The model under review builds one solid part; all positions refer to its coordinate system, in mm. A direction names the side the tool comes from. Coordinates: 2 decimals unless noted, no trailing zeros. Order: outer loops, then holes, each group sorted by start corner. A loop starts at its lowest first (then second) coordinate and runs counter-clockwise, first axis right, second up.
Autodesk Inventor part; units mm, degrees
ref_plane "YZ Plane" through (0, 0, 0) normal (1, 0, 0) x (0, 1, 0)
ref_plane "XZ Plane" through (0, 0, 0) normal (0, 1, 0) x (-1, 0, 0)
ref_plane "XY Plane" through (0, 0, 0) normal (0, 0, 1) x (1, 0, 0)
sketch "CONTOURS" plane through (0, 0, 0) normal (0, 0, 1) x (1, 0, 0)
  line L0 (1512.926, 262.3244) -> (1483.7011, 302.5491)
  arc A0 (1490.3116, 325.9808) -> (1483.7011, 302.5491) centre (1496.2408, 311.6597) ccw
  line L1 (1490.3116, 325.9808) -> (1515.055, 336.2252)
  arc A1 (1515.055, 336.2252) -> (1520.7765, 358.748) centre (1509.5083, 349.6224) ccw
  line L2 (1520.7765, 358.748) -> (1420.6454, 482.3882)
  arc A2 (1420.6454, 482.3882) -> (1397.875, 482.0914) centre (1409.3772, 473.2625) ccw
  line L3 (1397.875, 482.0914) -> (1387.5892, 468.6913)
  arc A3 (1362.754, 469.0184) -> (1387.5892, 468.6913) centre (1375.2938, 478.1291) ccw
  line L4 (1362.754, 469.0184) -> (1334.3843, 508.066)
  arc A4 (193.4245, 508.066) -> (1334.3843, 508.066) centre (763.9044, 1294.3771) ccw
  line L5 (193.4245, 508.066) -> (165.0547, 469.0184)
  arc A5 (165.0547, 469.0184) -> (171.943, 446.828) centre (176.7854, 460.4955) ccw
  line L6 (171.943, 446.828) -> (187.8658, 441.1866)
  arc A6 (195.6892, 418.1351) -> (187.8658, 441.1866) centre (182.6894, 426.5765) ccw
  line L7 (195.6892, 418.1351) -> (109.0426, 284.6979)
  arc A7 (84.2549, 283.0747) -> (109.0426, 284.6979) centre (96.0429, 293.1392) ccw
  line L8 (84.2549, 283.0747) -> (66.8658, 303.4414)
  arc A8 (66.8658, 303.4414) -> (44.1076, 302.5491) centre (55.8384, 294.0262) ccw
  line L9 (44.1076, 302.5491) -> (14.8827, 262.3244)
  arc A9 (14.8827, 262.3244) -> (1512.926, 262.3244) centre (763.9044, 1294.1149) ccw
sketch "HOLES" plane through (0, 0, 0) normal (0, 0, 1) x (1, 0, 0)
  line L0 (224.6944, 455.9957) -> (218.4625, 446.9313)
  arc A0 (212.9002, 445.9014) -> (218.4625, 446.9313) centre (215.1664, 449.1975) ccw
  line L1 (212.9002, 445.9014) -> (183.2349, 466.2968)
  arc A1 (182.205, 471.8591) -> (183.2349, 466.2968) centre (185.5011, 469.5929) ccw
  line L2 (182.205, 471.8591) -> (188.4369, 480.9234)
  arc A2 (193.9992, 481.9534) -> (188.4369, 480.9234) centre (191.733, 478.6573) ccw
  line L3 (193.9992, 481.9534) -> (223.6644, 461.558)
  arc A3 (224.6944, 455.9957) -> (223.6644, 461.558) centre (221.3983, 458.2619) ccw
  line L4 (87.0245, 255.754) -> (80.7926, 246.6896)
  arc A4 (75.2303, 245.6596) -> (80.7926, 246.6896) centre (77.4965, 248.9557) ccw
  line L5 (75.2303, 245.6596) -> (45.5651, 266.055)
  arc A5 (44.5351, 271.6173) -> (45.5651, 266.055) centre (47.8312, 269.3511) ccw
  line L6 (44.5351, 271.6173) -> (50.767, 280.6817)
  arc A6 (56.3293, 281.7117) -> (50.767, 280.6817) centre (54.0631, 278.4155) ccw
  line L7 (56.3293, 281.7117) -> (85.9946, 261.3163)
  arc A7 (87.0245, 255.754) -> (85.9946, 261.3163) centre (83.7284, 258.0201) ccw
  line L8 (1487.4439, 359.9016) -> (1478.716, 353.2066)
  arc A8 (1473.1076, 353.9459) -> (1478.716, 353.2066) centre (1476.2814, 356.3804) ccw
  line L9 (1473.1076, 353.9459) -> (1406.7666, 440.4321)
  arc A9 (1407.5058, 446.0405) -> (1406.7666, 440.4321) centre (1409.9404, 442.8667) ccw
  line L10 (1407.5058, 446.0405) -> (1416.2338, 452.7354)
  arc A10 (1421.8421, 451.9962) -> (1416.2338, 452.7354) centre (1418.6683, 449.5616) ccw
  line L11 (1421.8421, 451.9962) -> (1488.1832, 365.51)
  arc A11 (1487.4439, 359.9016) -> (1488.1832, 365.51) centre (1485.0094, 363.0754) ccw
sketch "LETTERS" plane through (0, 0, 0) normal (0, 0, 1) x (1, 0, 0)
  line L0 (221.0345, 299.5651) -> (214.0787, 303.3807)
  line L1 (214.0787, 303.3807) -> (223.8436, 320.6336)
  line L2 (223.8436, 320.6336) -> (229.7881, 317.2691)
  line L3 (232.463, 314.1509) -> (232.5322, 313.9591)
  line L4 (232.5322, 313.9591) -> (232.5968, 313.7631)
  line L5 (232.5968, 313.7631) -> (232.6568, 313.5633)
  line L6 (232.6568, 313.5633) -> (232.7121, 313.3597)
  line L7 (232.7121, 313.3597) -> (232.7625, 313.1525)
  line L8 (232.7625, 313.1525) -> (232.8082, 312.942)
  line L9 (232.8082, 312.942) -> (232.8489, 312.7282)
  line L10 (232.8489, 312.7282) -> (232.8846, 312.5116)
  line L11 (232.8846, 312.5116) -> (232.9153, 312.2921)
  line L12 (232.9153, 312.2921) -> (232.941, 312.0702)
  line L13 (232.941, 312.0702) -> (232.9616, 311.8459)
  line L14 (232.9616, 311.8459) -> (232.9772, 311.6196)
  line L15 (232.9772, 311.6196) -> (232.9877, 311.3915)
  line L16 (232.9877, 311.3915) -> (232.9931, 311.1618)
  line L17 (232.9931, 311.1618) -> (232.9936, 310.9307)
  line L18 (232.9936, 310.9307) -> (232.989, 310.6985)
  line L19 (232.989, 310.6985) -> (232.9795, 310.4654)
  line L20 (232.9795, 310.4654) -> (232.9651, 310.2317)
  line L21 (232.9651, 310.2317) -> (232.9458, 309.9975)
  line L22 (232.9458, 309.9975) -> (232.9218, 309.7632)
  line L23 (232.9218, 309.7632) -> (232.8931, 309.529)
  line L24 (232.8931, 309.529) -> (232.8598, 309.295)
  line L25 (232.8598, 309.295) -> (232.8219, 309.0616)
  line L26 (232.8219, 309.0616) -> (232.7797, 308.8289)
  line L27 (232.7797, 308.8289) -> (232.7331, 308.5971)
  line L28 (232.7331, 308.5971) -> (232.6823, 308.3664)
  line L29 (232.6823, 308.3664) -> (232.6274, 308.1371)
  line L30 (232.6274, 308.1371) -> (232.5686, 307.9094)
  line L31 (232.5686, 307.9094) -> (232.4396, 307.4592)
  line L32 (232.4396, 307.4592) -> (232.2964, 307.0174)
  line L33 (232.2964, 307.0174) -> (232.14, 306.585)
  line L34 (232.14, 306.585) -> (231.9716, 306.1633)
  line L35 (231.9716, 306.1633) -> (231.7923, 305.7532)
  line L36 (231.6033, 305.3555) -> (231.402, 304.9639)
  line L37 (231.402, 304.9639) -> (231.185, 304.5725)
  line L38 (231.185, 304.5725) -> (230.9521, 304.1826)
  line L39 (230.9521, 304.1826) -> (230.7035, 303.7959)
  line L40 (230.7035, 303.7959) -> (230.4394, 303.4138)
  line L41 (230.4394, 303.4138) -> (230.16, 303.038)
  line L42 (230.16, 303.038) -> (230.0147, 302.853)
  line L43 (230.0147, 302.853) -> (229.8658, 302.6702)
  line L44 (229.8658, 302.6702) -> (229.7134, 302.4898)
  line L45 (229.7134, 302.4898) -> (229.5575, 302.3121)
  line L46 (229.5575, 302.3121) -> (229.3982, 302.1372)
  line L47 (229.3982, 302.1372) -> (229.2357, 301.9654)
  line L48 (229.2357, 301.9654) -> (229.07, 301.7969)
  line L49 (229.07, 301.7969) -> (228.9013, 301.6319)
  line L50 (228.9013, 301.6319) -> (228.7297, 301.4705)
  line L51 (228.7297, 301.4705) -> (228.5554, 301.3131)
  line L52 (228.5554, 301.3131) -> (228.3784, 301.1597)
  line L53 (228.3784, 301.1597) -> (228.1989, 301.0107)
  line L54 (228.1989, 301.0107) -> (228.0172, 300.8661)
  line L55 (228.0172, 300.8661) -> (227.8333, 300.7261)
  line L56 (227.8333, 300.7261) -> (227.6474, 300.591)
  line L57 (227.6474, 300.591) -> (227.4598, 300.4608)
  line L58 (227.4598, 300.4608) -> (227.2705, 300.3358)
  line L59 (227.2705, 300.3358) -> (227.0798, 300.2161)
  line L60 (227.0798, 300.2161) -> (226.8878, 300.1017)
  line L61 (226.8878, 300.1017) -> (226.6948, 299.9929)
  line L62 (229.9244, 317.199) -> (230.0598, 317.1238)
  line L63 (230.0598, 317.1238) -> (230.1939, 317.0436)
  line L64 (230.1939, 317.0436) -> (230.3268, 316.9582)
  line L65 (230.3268, 316.9582) -> (230.4581, 316.8676)
  line L66 (230.4581, 316.8676) -> (230.5878, 316.7718)
  line L67 (230.5878, 316.7718) -> (230.7158, 316.6707)
  line L68 (231.7923, 305.7532) -> (231.6033, 305.3555)
  line L69 (230.7158, 316.6707) -> (230.8417, 316.5642)
  line L70 (230.8417, 316.5642) -> (230.9656, 316.4525)
  line L71 (230.9656, 316.4525) -> (231.0872, 316.3353)
  line L72 (231.0872, 316.3353) -> (231.2064, 316.2128)
  line L73 (231.2064, 316.2128) -> (231.3229, 316.085)
  line L74 (221.173, 299.4993) -> (221.0345, 299.5651)
  line L75 (231.3229, 316.085) -> (231.4367, 315.9518)
  line L76 (231.4367, 315.9518) -> (231.5476, 315.8134)
  line L77 (231.5476, 315.8134) -> (231.6554, 315.6696)
  line L78 (231.6554, 315.6696) -> (231.76, 315.5207)
  line L79 (229.7881, 317.2691) -> (229.9244, 317.199)
  line L80 (231.76, 315.5207) -> (231.8612, 315.3665)
  line L81 (231.8612, 315.3665) -> (231.9589, 315.2073)
  line L82 (231.9589, 315.2073) -> (232.0529, 315.0431)
  line L83 (232.0529, 315.0431) -> (232.1431, 314.874)
  line L84 (232.1431, 314.874) -> (232.2293, 314.7001)
  line L85 (232.2293, 314.7001) -> (232.3115, 314.5216)
  line L86 (232.3115, 314.5216) -> (232.3894, 314.3384)
  line L87 (232.3894, 314.3384) -> (232.463, 314.1509)
  line L88 (221.3149, 299.4374) -> (221.173, 299.4993)
  line L89 (221.4601, 299.3795) -> (221.3149, 299.4374)
  line L90 (221.6085, 299.3258) -> (221.4601, 299.3795)
  line L91 (221.7603, 299.2764) -> (221.6085, 299.3258)
  line L92 (221.9152, 299.2315) -> (221.7603, 299.2764)
  line L93 (222.0732, 299.1913) -> (221.9152, 299.2315)
  line L94 (222.2342, 299.1558) -> (222.0732, 299.1913)
  line L95 (222.3983, 299.1252) -> (222.2342, 299.1558)
  line L96 (222.5652, 299.0997) -> (222.3983, 299.1252)
  line L97 (222.7348, 299.0794) -> (222.5652, 299.0997)
  line L98 (222.9072, 299.0644) -> (222.7348, 299.0794)
  line L99 (223.0821, 299.0548) -> (222.9072, 299.0644)
  line L100 (223.2595, 299.0507) -> (223.0821, 299.0548)
  line L101 (223.4391, 299.0523) -> (223.2595, 299.0507)
  line L102 (223.621, 299.0597) -> (223.4391, 299.0523)
  line L103 (223.8049, 299.0728) -> (223.621, 299.0597)
  line L104 (223.9907, 299.0918) -> (223.8049, 299.0728)
  line L105 (224.1783, 299.1168) -> (223.9907, 299.0918)
  line L106 (224.3674, 299.1478) -> (224.1783, 299.1168)
  line L107 (224.5579, 299.1849) -> (224.3674, 299.1478)
  line L108 (224.7497, 299.228) -> (224.5579, 299.1849)
  line L109 (224.9425, 299.2773) -> (224.7497, 299.228)
  line L110 (225.1362, 299.3327) -> (224.9425, 299.2773)
  line L111 (225.3306, 299.3942) -> (225.1362, 299.3327)
  line L112 (225.5256, 299.4618) -> (225.3306, 299.3942)
  line L113 (225.7208, 299.5354) -> (225.5256, 299.4618)
  line L114 (225.9161, 299.6151) -> (225.7208, 299.5354)
  line L115 (226.1114, 299.7008) -> (225.9161, 299.6151)
  line L116 (226.3064, 299.7923) -> (226.1114, 299.7008)
  line L117 (226.5009, 299.8898) -> (226.3064, 299.7923)
  line L118 (226.6948, 299.9929) -> (226.5009, 299.8898)
extrude "Extrusion1" add sketch "CONTOURS" along normal blind 18
extrude "Extrusion2" cut sketch "HOLES" along normal blind 18
properties part number "Platform D3" material "Wood (Birch)"
(1) We need section C-C, the plane x = 919.5. Write out the cut boundary in (y, z).
A:
outline: (28.64, 0) - (335.46, 0) - (335.46, 18) - (28.64, 18) - close
(2) Wall thickness on probe 1 along X at (y, z) = (263, 14.75); probe 2 along Y at (x, z) = (467.5, 10.25); probe 3 along X at (y, z) = (212, 7): over which ranges is each line inside the solid? List them lowest first.
A:
probe 1: x = 15.37 to 50.01, 83.55 to 1512.44
probe 2: y = 54.05 to 369.24
probe 3: x = 89.63 to 1438.18
(3) Machinability: for faces 5 (the face through (179.44, 488.82, 8.87)), 6 (the face through (152.97, 352.35, 8.87)), 7 (the face through (1348.768, 488.269, 8.874)), which of the approach directions +Z, -Z, +X, -X, +Y, -Y give a long, thin tool a straight path to every point of the face, cutting with its end or side? Answer none if there is none.
A:
face 5: +Z, -Z, -X, +Y
face 6: +Z, -Z
face 7: +Z, -Z, +Y
(4) Draft analysis for pull direction X (two halves, no side actions). For faces 1 (the face through (775.113, 19.164, 8.874)), 2 (the face through (1498.518, 282.155, 8.874)), 3 (the face through (772.441, 322.956, 8.874)), 4 (the face through (759, 213, 0)), state which applies: released by +X, released by -X, zero draft, split by the parting line, or undercut.
A:
face 1: split by the parting line
face 2: released by +X
face 3: undercut
face 4: zero draft
(5) For pin 1 Ø8 at (x, z) = (1008.5, 11) entering from +Y; pin 2 Ø6 at (x, z) = (1144.5, 10) entering from -Y; pin 3 Ø10 at (x, z) = (279, 6.5) entering from +Y, all flat-tipped, find the tip position at first contact; note any pin that passes through.
A:
pin 1: stops at y = 355.26
pin 2: stops at y = 76.31
pin 3: stops at y = 455.49
(6) We need section B-B, the plane z = 13.5. Count the separate pieces of the cut face and the enclosed holes in it, and give its area (3 significant figures).
A:
separate pieces: 1
enclosed holes: 3
area: 424,000 mm2
(7) We need section D-D, the plane y = 152.5. Write out the cut boundary in (x, z), and give its area (3 significant figures).
A:
outline: (196.15, 0) - (1331.65, 0) - (1331.65, 18) - (196.15, 18) - close
area: 20,400 mm2
(8) We need section A-A, the plane y = 400. Write out the cut boundary in (x, z).
A:
outline: (183.91, 0) - (384.67, 0) - (384.67, 18) - (183.91, 18) - close; (1143.14, 0) - (1437.78, 0) - (1437.78, 18) - (1143.14, 18) - close; (1461.73, 0) - (1487.37, 0) - (1487.37, 18) - (1461.73, 18) - close
